Here's how the part is built. I have some questions about the finished solid (model axes, mm). Give positions to 0.01 mm unless a question says otherwise; leave off trailing zeros. Order: outer loops, then holes, each group sorted by start corner. A loop starts at its lowest first (then second) coordinate and runs counter-clockwise, first axis right, second up. Notation, with made-up numbers: (-2.75, 24) - (39.25, 24) arc R22 cw to (39.25, 61) - close; hole circle Ø10 at (-14, -21). An arc over 180 degrees is marked (long way). One line per question, with ' | ' between items.
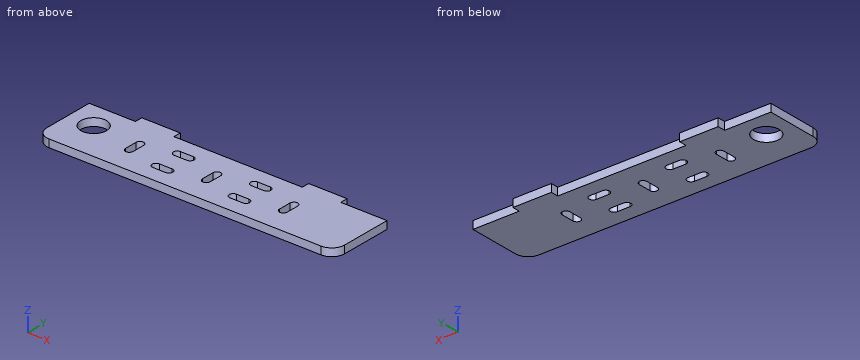
from build123d import *

# Parameters (mm, degrees)
BOSS_EXTRUDE1_DEPTH = 3
SKETCH3_R           = 5
CUT_EXTRUDE2_DEPTH  = 64.229739838
CUT_EXTRUDE3_DEPTH  = 64.229739838


with BuildPart() as part:
    # Sketch1 → Boss-Extrude1 (new body)
    with BuildSketch(Plane.XY):
        with BuildLine():
            Line((-25, 0), (25, 0))
            Line((25, 0), (25, 3))
            Line((25, 3), (40, 3))
            Line((40, 3), (40, 0))
            Line((40, 0), (58, 0))
            Line((58, 0), (58, -20))
            ThreePointArc((58, -20), (56.535533906, -23.535533906), (53, -25))
            Line((53, -25), (-53, -25))
            ThreePointArc((-53, -25), (-56.535533906, -23.535533906), (-58, -20))
            Line((-58, -20), (-58, 0))
            Line((-58, 0), (-40, 0))
            Line((-40, 0), (-40, 3))
            Line((-40, 3), (-25, 3))
            Line((-25, 3), (-25, 0))
        make_face()
    extrude(amount=BOSS_EXTRUDE1_DEPTH)

    # Sketch3 → Cut-Extrude2 (cut, through all)
    with BuildSketch(Plane(origin=(0, 0, 0), x_dir=(-1, 0, 0), z_dir=(0, 0, -1))):
        with Locations((48, -10)):
            Circle(SKETCH3_R)
    extrude(amount=-CUT_EXTRUDE2_DEPTH, mode=Mode.SUBTRACT)

    # Sketch4 → Cut-Extrude3 (cut, through all)
    with BuildSketch(Plane(origin=(0, 0, 0), x_dir=(-1, 0, 0), z_dir=(0, 0, -1))):
        with BuildLine():
            Line((-28.5, -10), (-28.5, -15))
            ThreePointArc((-28.5, -15), (-30, -16.5), (-31.5, -15))
            Line((-31.5, -15), (-31.5, -10))
            ThreePointArc((-31.5, -10), (-30, -8.5), (-28.5, -10))
        make_face()
        with BuildLine():
            Line((-17.5, -6), (-12.5, -6))
            ThreePointArc((-12.5, -6), (-11, -7.5), (-12.5, -9))
            Line((-12.5, -9), (-17.5, -9))
            ThreePointArc((-17.5, -9), (-19, -7.5), (-17.5, -6))
        make_face()
        with BuildLine():
            Line((-1.5, -15), (-1.5, -10))
            ThreePointArc((-1.5, -10), (0, -8.5), (1.5, -10))
            Line((1.5, -10), (1.5, -15))
            ThreePointArc((1.5, -15), (0, -16.5), (-1.5, -15))
        make_face()
        with BuildLine():
            Line((28.5, -15), (28.5, -10))
            ThreePointArc((28.5, -10), (30, -8.5), (31.5, -10))
            Line((31.5, -10), (31.5, -15))
            ThreePointArc((31.5, -15), (30, -16.5), (28.5, -15))
        make_face()
        with BuildLine():
            Line((12.5, -6), (17.5, -6))
            ThreePointArc((17.5, -6), (19, -7.5), (17.5, -9))
            Line((17.5, -9), (12.5, -9))
            ThreePointArc((12.5, -9), (11, -7.5), (12.5, -6))
        make_face()
        with BuildLine():
            Line((12.5, -16), (17.5, -16))
            ThreePointArc((17.5, -16), (19, -17.5), (17.5, -19))
            Line((17.5, -19), (12.5, -19))
            ThreePointArc((12.5, -19), (11, -17.5), (12.5, -16))
        make_face()
        with BuildLine():
            Line((-17.5, -16), (-12.5, -16))
            ThreePointArc((-12.5, -16), (-11, -17.5), (-12.5, -19))
            Line((-12.5, -19), (-17.5, -19))
            ThreePointArc((-17.5, -19), (-19, -17.5), (-17.5, -16))
        make_face()
    extrude(amount=-CUT_EXTRUDE3_DEPTH, mode=Mode.SUBTRACT)


solid = part.part
1) I want a section at C-C (z = 2). State how many separate pieces and enclosed holes the cut face has, plus the area to 3 significant figures.
Model answer:
separate pieces: 1 | enclosed holes: 8 | area: 2,750 mm2
2) I want a section at D-D (x = -48). List the corners of the cut face in (y, z) for me, plus the area to 3 significant figures.
Model answer:
outline: (-25, 0) - (-15, 0) - (-15, 3) - (-25, 3) - close; (-5, 0) - (0, 0) - (0, 3) - (-5, 3) - close | area: 45.0 mm2
3) Please list where these lines run through material, in increasing order: L1, parallel to X at y = -12.5, z = 1.9; L2, parallel to X at y = -18.75, z = 1.75; L3, parallel to X at y = -13.5, z = 2.4.
Model answer:
L1: x = -58 to -52.33, -43.67 to -31.5, -28.5 to -1.5, 1.5 to 28.5, 31.5 to 58 | L2: x = -58 to -18.33, -11.67 to 11.67, 18.33 to 58 | L3: x = -58 to -51.57, -44.43 to -31.5, -28.5 to -1.5, 1.5 to 28.5, 31.5 to 58
4) I want a section at A-A (x = -30). List the corners of the cut face in (y, z) for me.
Model answer:
outline: (-25, 0) - (-16.5, 0) - (-16.5, 3) - (-25, 3) - close; (-8.5, 0) - (3, 0) - (3, 3) - (-8.5, 3) - close
5) I want a section at B-B (y = -17.5). List the corners of the cut face in (x, z) for me, plus the area to 3 significant figures.
Model answer:
outline: (-58, 0) - (-19, 0) - (-19, 3) - (-58, 3) - close; (-11, 0) - (11, 0) - (11, 3) - (-11, 3) - close; (19, 0) - (58, 0) - (58, 3) - (19, 3) - close | area: 300 mm2
6) I'm going to push flat-ended pins straight in: P1, Ø0.9, axis at x = 49, z = 2, coming from the +Y side; P2, Ø0.9, axis at y = 1, z = 1.5, coming from the +X side. Where does each tip first touch, or does it pass through?
Model answer:
P1: stops at y = 0 | P2: stops at x = 40
